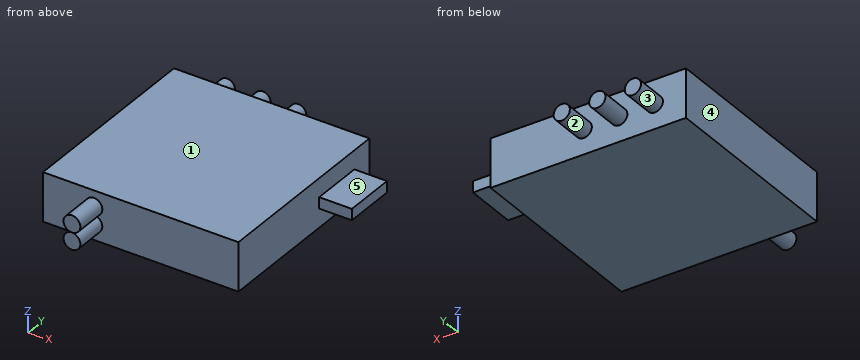
from build123d import *

# Parameters (mm, degrees)
SKETCH1_W           = 52.38
SKETCH1_H           = 13.01
BOSS_EXTRUDE1_DEPTH = 52.2
SKETCH2_R           = 2.26
BOSS_EXTRUDE6_DEPTH = 8.75
SKETCH3_R           = 2.175
BOSS_EXTRUDE7_DEPTH = 8.75
SKETCH4_W           = 3
SKETCH4_H           = 14
BOSS_EXTRUDE8_DEPTH = 8.75


with BuildPart() as part:
    # Sketch1 → Boss-Extrude1 (new body)
    with BuildSketch(Plane(origin=(0, 0, 0), x_dir=(1, 0, 0), z_dir=(0, 1, 0))):
        Rectangle(SKETCH1_W, SKETCH1_H)
    extrude(amount=BOSS_EXTRUDE1_DEPTH)

    # Sketch2 → Boss-Extrude6 (add)
    with BuildSketch(Plane(origin=(0, 0, 0), x_dir=(-1, 0, 0), z_dir=(0, -1, 0))):
        with Locations((12.55, -2.27)):
            Circle(SKETCH2_R)
        with Locations((12.55, 2.27)):
            Circle(SKETCH2_R)
    extrude(amount=BOSS_EXTRUDE6_DEPTH)

    # Sketch3 → Boss-Extrude7 (add)
    with BuildSketch(Plane(origin=(0, 52.2, 0), x_dir=(1, 0, 0), z_dir=(0, 1, 0))):
        with Locations((-17.825, 0)):
            Circle(SKETCH3_R)
        with Locations((-8.295, 0)):
            Circle(SKETCH3_R)
        with Locations((1.235, 0)):
            Circle(SKETCH3_R)
    extrude(amount=BOSS_EXTRUDE7_DEPTH)

    # Sketch4 → Boss-Extrude8 (add)
    with BuildSketch(Plane(origin=(26.19, 0, 0), x_dir=(0, 0, -1), z_dir=(1, 0, 0))):
        with Locations((0, 39.2)):
            Rectangle(SKETCH4_W, SKETCH4_H)
    extrude(amount=BOSS_EXTRUDE8_DEPTH)


solid = part.part
Source: CAD feature listing. Evaluate the final solid. Frame: model axes, mm. Face numbers are marked on the shaded views. A direction names the side the tool comes from. Give positions to 0.01 mm unless a question says otherwise; leave off trailing zeros. Write each loop counter-clockwise with the first axis right and the second up, starting at its lowest first coordinate (ties: lowest second). Pieces come first, ordered by that corner, then holes. Notation, with made-up numbers: (52.25, 29.25) - (63.25, 29.25) arc R19 ccw to (63.25, 40.25) - close; hole circle Ø10 at (30.5, 21). An arc over 180 degrees is marked (long way). Write item = value, one per line. Start each with the question number.
Q1. Cut plane A-A, the plane y = 39.5. Return loops of the section in (x, z) (3 decimals), then the cut area to 3 significant figures.
Q2. Material intervals for probe 1 along X at (y, z) = (28, 4.25); probe 2 along Y at (x, z) = (18, 0); probe 3 along Y at (x, z) = (-18, -1.5), sorted ascending.
Q3. Cut plane C-C, the plane z = 3.5. Return loops of the section in (x, y), then the cut area to 3 significant figures.
Q4. Reachability of the marked faces 1 and 2 from +Z, -Z, +X, -X, +Y, -Y: full face, straight path, thin tool, end or side. Return the list, or none.
Q5. Cut plane B-B, the plane x = -12.55. Return loops of the section in (y, z) (3 decimals).
Q6. Pin query (flat end, axial travel): pin 1 Ø5 at (y, z) = (38.5, -4.5) entering from +X; pin 2 Ø7 at (x, y) = (32.5, 40.5) entering from -Z; pin 3 Ø0.9 at (x, z) = (31, 0) entering from -Y. Return the tip coordinate at first contact, or that it passes through.
Q7. Draft query along X for the marked faces 3, 4 and 5. Return one class per face: +X half, -X half, draft (parallel to the pull), parting line (faces both ways), or undercut.
Q8. Cut plane D-D, the plane x = 31. Return loops of the section in (y, z), then the cut area to 3 significant figures.
Computed values:
q1.outline = (-26.19, -6.505) - (26.19, -6.505) - (26.19, -1.5) - (34.94, -1.5) - (34.94, 1.5) - (26.19, 1.5) - (26.19, 6.505) - (-26.19, 6.505) - close
q1.area = 708 mm²
q2.probe_1 = -26.19 to 26.19
q2.probe_2 = 0 to 52.2
q2.probe_3 = 0 to 60.95
q3.outline = (-26.19, 0) - (-14.45, 0) - (-14.45, -8.75) - (-10.65, -8.75) - (-10.65, 0) - (26.19, 0) - (26.19, 52.2) - (-26.19, 52.2) - close
q3.area = 2,770 mm²
q4.face_1 = +Z, +X, -X, +Y, -Y
q4.face_2 = +Y
q5.outline = (-8.75, -4.53) - (0, -4.53) - (0, -6.505) - (52.2, -6.505) - (52.2, 6.505) - (0, 6.505) - (0, 4.53) - (-8.75, 4.53) - (-8.75, 0.01) - (0, 0.01) - (0, -0.01) - (-8.75, -0.01) - close
q6.pin_1 = 26.19
q6.pin_2 = -1.5
q6.pin_3 = 32.2
q7.face_3 = undercut
q7.face_4 = -X half
q7.face_5 = draft
q8.outline = (32.2, -1.5) - (46.2, -1.5) - (46.2, 1.5) - (32.2, 1.5) - close
q8.area = 42.0 mm²
